from build123d import *

# Parameters (mm, degrees)
SKETCH_1_W          = 55
SKETCH_1_H          = 55
EXTRUDE_1_DEPTH     = 10
SKETCH_2_W          = 52
SKETCH_2_H          = 52
CUT_EXTRUDE_1_DEPTH = 8
FILLET_1_R          = 2
SKETCH_3_R          = 2.5
EXTRUDE_2_DEPTH     = 4
SKETCH_5_R          = 1.1
CUT_EXTRUDE_2_DEPTH = 4
EXTRUDE_4_DEPTH     = 4
EXTRUDE_6_DEPTH     = 4


with BuildPart() as part:
    # 草图1 → 凸台-拉伸1 (new body)
    with BuildSketch(Plane.XY):
        Rectangle(SKETCH_1_W, SKETCH_1_H)
    extrude(amount=EXTRUDE_1_DEPTH)

    # 草图2 → 切除-拉伸1 (cut)
    with BuildSketch(Plane.XY.offset(10)):
        Rectangle(SKETCH_2_W, SKETCH_2_H)
    extrude(amount=-CUT_EXTRUDE_1_DEPTH, mode=Mode.SUBTRACT)

    # 圆角1
    fillet_1_edges = [part.edges().sort_by_distance(p)[0] for p in [
        (0, -27.5, 0),
        (-27.5, 0, 0),
        (0, 27.5, 0),
        (27.5, 0, 0),
    ]]
    fillet(fillet_1_edges, radius=FILLET_1_R)

    # 草图3 → 凸台-拉伸2 (add)
    with BuildSketch(Plane.XY.offset(2)):
        with Locations((-22.5, 22.5)):
            Circle(SKETCH_3_R)
        with Locations((22.5, 22.5)):
            Circle(SKETCH_3_R)
        with Locations((-22.5, -22.5)):
            Circle(SKETCH_3_R)
        with Locations((22.5, -22.5)):
            Circle(SKETCH_3_R)
    extrude(amount=EXTRUDE_2_DEPTH)

    # 草图5 → 切除-拉伸2 (cut)
    with BuildSketch(Plane.XY.offset(6)):
        with Locations((-22.5, -22.5)):
            Circle(SKETCH_5_R)
        with Locations((22.5, -22.5)):
            Circle(SKETCH_5_R)
        with Locations((-22.5, 22.5)):
            Circle(SKETCH_5_R)
        with Locations((22.5, 22.5)):
            Circle(SKETCH_5_R)
    extrude(amount=-CUT_EXTRUDE_2_DEPTH, mode=Mode.SUBTRACT)

    # 草图6 → 凸台-拉伸4 (add)
    with BuildSketch(Plane.XY.offset(2)):
        with BuildLine():
            ThreePointArc((-22.5, 20), (-25, 22.5), (-22.5, 25))
            Line((-22.5, 25), (-26, 25))
            Line((-26, 25), (-26, 20))
            Line((-26, 20), (-22.5, 20))
        make_face()
    extrude(amount=EXTRUDE_4_DEPTH)

    # 草图13 → 凸台-拉伸6 (add)
    with BuildSketch(Plane.XY.offset(2)):
        with BuildLine():
            ThreePointArc((-22.5, 25), (-20.732233047, 24.267766953), (-20, 22.5))
            Line((-20, 22.5), (-20, 26))
            Line((-20, 26), (-26, 26))
            Line((-26, 26), (-26, 25))
            Line((-26, 25), (-22.5, 25))
        make_face()
        with BuildLine():
            ThreePointArc((-20, -22.5), (-24.267766953, -24.267766953), (-22.5, -20))
            Line((-22.5, -20), (-26, -20))
            Line((-26, -20), (-26, -26))
            Line((-26, -26), (-20, -26))
            Line((-20, -26), (-20, -22.5))
        make_face()
        with BuildLine():
            Line((26, -20), (22.5, -20))
            ThreePointArc((22.5, -20), (24.267766953, -24.267766953), (20, -22.5))
            Line((20, -22.5), (20, -26))
            Line((20, -26), (26, -26))
            Line((26, -26), (26, -20))
        make_face()
        with BuildLine():
            Line((20, 26), (20, 22.5))
            ThreePointArc((20, 22.5), (24.267766953, 24.267766953), (22.5, 20))
            Line((22.5, 20), (26, 20))
            Line((26, 20), (26, 26))
            Line((26, 26), (20, 26))
        make_face()
    extrude(amount=EXTRUDE_6_DEPTH)


solid = part.part
Work out the finished part from the listing and answer in its coordinate system (mm). A direction names the side the tool comes from. Round coordinates to 2 decimals unless told otherwise and drop trailing zeros. Write each loop counter-clockwise with the first axis right and the second up, starting at its lowest first coordinate (ties: lowest second). Pieces come first, ordered by that corner, then holes.
1) Straight lines are drawn through the part: line 1 (Y direction, x = 22.5, z = 4.4); line 2 (Y direction, x = -13.5, z = 3). For each, find the intervals that lie inside material, in ascending order.
2) A tool of negligible diameter and unlimited length cuts with its end or side. For faces 4 (the flat face through (24, -20, 4)), 5 (the flat face through (27.5, 0, 6)), from which of +Z, -Z, +X, -X, +Y, -Y can it reach the whole face along a straight path? Write none if from no direction.
3) The mould has two halves that part along Y. Classify faces 1 (the cylindrical face through (20.752, -20.713, 3.972)), 2 (the cylindrical face through (0.39, 26.93, 0.6)), 3 (the cylindrical face through (-26.93, 0.39, 0.6)): pulls with the +Y half, pulls with the -Y half, needs draft (parallel to the pull), parting line crosses it, or undercut.
4) Given pin 1 Ø1.1 at (x, y) = (-22.5, 23) entering from +Z; pin 2 Ø3 at (x, y) = (22.5, 22.5) entering from +Z, each flat-ended and moving along its own axis, determine where each tip first touches the part or whether it passes through.
5) A cutting plane is placed at B-B (y = -18.5). Give the vertices of the cut face in (x, z).
6) A cutting plane is placed at C-C (z = 7.5). Give the vertices of the cut face in (x, y), plus the area to 3 significant figures.
7) A cutting plane is placed at A-A (z = 4.25). Give the vertices of the cut face in (x, y), plus the area to 3 significant figures.
Completed:
1. line 1: y = -27.5 to -23.6, -21.4 to -20, 20 to 21.4, 23.6 to 27.5
1. line 2: y = -27.5 to -26, 26 to 27.5
2. face 4: +Z
2. face 5: +Z, -Z, +X, +Y, -Y
3. face 1: undercut
3. face 2: pulls with the +Y half
3. face 3: needs draft
4. pin 1: stops at z = 2
4. pin 2: stops at z = 6
5. outline: (-27.5, 2) arc R2 ccw to (-25.5, 0) - (25.5, 0) arc R2 ccw to (27.5, 2) - (27.5, 10) - (26, 10) - (26, 2) - (-26, 2) - (-26, 10) - (-27.5, 10) - close
6. outline: (-27.5, -27.5) - (27.5, -27.5) - (27.5, 27.5) - (-27.5, 27.5) - close; hole (-26, -26) - (26, -26) - (26, 26) - (-26, 26) - close
6. area: 321 mm2
7. outline: (-27.5, -27.5) - (27.5, -27.5) - (27.5, 27.5) - (-27.5, 27.5) - close; hole (-26, -20) - (-22.5, -20) arc R2.5 cw to (-20, -22.5) - (-20, -26) - (20, -26) - (20, -22.5) arc R2.5 cw to (22.5, -20) - (26, -20) - (26, 20) - (22.5, 20) arc R2.5 cw to (20, 22.5) - (20, 26) - (-20, 26) - (-20, 22.5) arc R2.5 cw to (-22.5, 20) - (-26, 20) - close; hole circle Ø2.2 at (-22.5, -22.5); hole circle Ø2.2 at (-22.5, 22.5); hole circle Ø2.2 at (22.5, -22.5); hole circle Ø2.2 at (22.5, 22.5)
7. area: 444 mm2
